Build history of the part. All positions in model axes, mm. Round coordinates to 2 decimals unless told otherwise and drop trailing zeros. Write each loop counter-clockwise with the first axis right and the second up, starting at its lowest first coordinate (ties: lowest second). Pieces come first, ordered by that corner, then holes.
1) Wall check: probe 1 along Z at (x, y) = (1.75, 0); probe 2 along Z at (x, y) = (4, 3); probe 3 along Y at (x, z) = (3.5, -3). Give the ranges that are in metal, low to high.
2) Saw through at D-D (y = -4.5). Write the cut outline in (x, z).
3) Pull direction Z, two halves, no side cores. Call faces 1 (the flat face through (3, 0, 6.495)), 2 (the flat face through (3.204, -5.651, -3.202)), 3 (the cylindrical face through (3.204, -0.867, 3.905)): +Z half, -Z half, draft (parallel to the pull), parting line (faces both ways), or undercut.
4) Saw through at A-A (x = 5.5). Write the cut outline in (y, z).
5) Saw through at C-C (z = -0.5). Write the cut outline in (x, y), plus the area to 3 significant figures.
6) Saw through at B-B (y = 0). Write the cut outline in (x, z), plus the area to 3 significant figures.
7) Flat gauge pins, fed straight in: pin 1 (3 mm diameter, centred on x = 5, y = 6, fed in from +Z); pin 2 (2 mm diameter, centred on x = 6, z = 3.5, fed in from -Y); pin 3 (1.5 mm diameter, centred on x = 3, z = 5, fed in from -Y). Where does each tip first touch, or does it go through?
Autodesk Inventor part; units mm, degrees
ref_plane "YZ Plane" through (0, 0, 0) normal (1, 0, 0) x (0, 1, 0)
ref_plane "XZ Plane" through (0, 0, 0) normal (0, 1, 0) x (-1, 0, 0)
ref_plane "XY Plane" through (0, 0, 0) normal (0, 0, 1) x (1, 0, 0)
sketch "スケッチ1" plane through (0, 0, 0) normal (1, 0, 0) x (0, 1, 0)
  circle A0 centre (0, 0) radius 7.5
  line L0 (7.5, 0) -> (3.75, 6.4952)
  line L1 (3.75, 6.4952) -> (-3.75, 6.4952)
  line L2 (-3.75, 6.4952) -> (-7.5, 0)
  line L3 (-7.5, 0) -> (-3.75, -6.4952)
  line L4 (-3.75, -6.4952) -> (3.75, -6.4952)
  line L5 (3.75, -6.4952) -> (7.5, 0)
  circle A1 centre (0, 0) radius 4
  point P0 (3.75, 6.4952)
  point P1 (-3.75, -6.4952)
  dimension "d0" = 15
  dimension "d3" = 360
  dimension "d5" = 8
extrude "押し出し1" add sketch "スケッチ1" along normal blind 6.5 contours L5 L4 L3 L2 L1 L0
properties part number "8min-nut" material "アルミニウム 6061"
Evaluation:
1. probe 1: z = -6.5 to -4, 4 to 6.5
1. probe 2: z = -6.5 to -2.65, 2.65 to 6.5
1. probe 3: y = -5.77 to -2.65, 2.65 to 5.77
2. outline: (0, -5.2) - (6.5, -5.2) - (6.5, 5.2) - (0, 5.2) - close
3. face 1: +Z half
3. face 2: -Z half
3. face 3: undercut
4. outline: (-7.5, 0) - (-3.75, -6.5) - (3.75, -6.5) - (7.5, 0) - (3.75, 6.5) - (-3.75, 6.5) - close; hole circle Ø8 at (0, 0)
5. outline: (0, -7.21) - (6.5, -7.21) - (6.5, -3.97) - (0, -3.97) - close; (0, 3.97) - (6.5, 3.97) - (6.5, 7.21) - (0, 7.21) - close
5. area: 42.2 mm2
6. outline: (0, -6.5) - (6.5, -6.5) - (6.5, -4) - (0, -4) - close; (0, 4) - (6.5, 4) - (6.5, 6.5) - (0, 6.5) - close
6. area: 32.4 mm2
7. pin 1: stops at z = 5.2
7. pin 2: stops at y = -6.06
7. pin 3: stops at y = -5.05
